```python
from build123d import *

# Parameters (mm, degrees)
SKETCH_1_W          = 40
SKETCH_1_H          = 37.5
EXTRUDE_1_DEPTH     = 19.9
SKETCH_2_W          = 7
SKETCH_2_H          = 19.9
EXTRUDE_2_DEPTH     = 2.5
CUT_EXTRUDE_1_DEPTH = 43.995581168


with BuildPart() as part:
    # 草图1 → 凸台-拉伸1 (new body)
    with BuildSketch(Plane.XY):
        Rectangle(SKETCH_1_W, SKETCH_1_H)
    extrude(amount=EXTRUDE_1_DEPTH)

    # 草图2 → 凸台-拉伸2 (add)
    with BuildSketch(Plane(origin=(0, 8.15, 0), x_dir=(-1, 0, 0), z_dir=(0, -1, 0))):
        with Locations((23.5, -9.95)):
            Rectangle(SKETCH_2_W, SKETCH_2_H)
        with Locations((-23.5, -9.95)):
            Rectangle(SKETCH_2_W, SKETCH_2_H)
    extrude(amount=EXTRUDE_2_DEPTH)

    # 草图3 → 切除-拉伸1 (cut, through all)
    with BuildSketch(Plane(origin=(0, 8.15, 0), x_dir=(1, 0, 0), z_dir=(0, 1, 0))):
        with BuildLine():
            Line((27, -15.9), (26.315564437, -15.9))
            ThreePointArc((26.315564437, -15.9), (22.05, -14.9), (26.315564437, -13.9))
            Line((26.315564437, -13.9), (27, -13.9))
            Line((27, -13.9), (27, -15.9))
        make_face()
        with BuildLine():
            Line((27, -6), (26.315564437, -6))
            ThreePointArc((26.315564437, -6), (22.05, -5), (26.315564437, -4))
            Line((26.315564437, -4), (27, -4))
            Line((27, -4), (27, -6))
        make_face()
        with BuildLine():
            Line((-27, -15.9), (-27, -13.9))
            Line((-27, -13.9), (-26.315564437, -13.9))
            ThreePointArc((-26.315564437, -13.9), (-22.05, -14.9), (-26.315564437, -15.9))
            Line((-26.315564437, -15.9), (-27, -15.9))
        make_face()
        with BuildLine():
            Line((-27, -4), (-27, -6))
            Line((-27, -6), (-26.315564437, -6))
            ThreePointArc((-26.315564437, -6), (-22.05, -5), (-26.315564437, -4))
            Line((-26.315564437, -4), (-27, -4))
        make_face()
    extrude(amount=-CUT_EXTRUDE_1_DEPTH, mode=Mode.SUBTRACT)


solid = part.part
```
Could you check a few things on this model? Use its own coordinates, in mm. A direction names the side the tool comes from. Coordinates: 2 decimals unless noted, no trailing zeros. Write each loop counter-clockwise with the first axis right and the second up, starting at its lowest first coordinate (ties: lowest second). Pieces come first, ordered by that corner, then holes. Notation, with made-up numbers: (45, 54.25) -> (104, 54.25) arc R24 cw to (104, 91.25) -> close; hole circle Ø2 at (1.5, -29.75). An arc over 180 degrees is marked (long way). Return JSON: item names as keys, results as strings.
(1) Imagine slicing it at A-A, the plane x = -24.3. Please give me the cut outline in (y, z).
Numbers:
{"outline": "(5.65, 0) -> (8.15, 0) -> (8.15, 2.75) -> (5.65, 2.75) -> close; (5.65, 7.25) -> (8.15, 7.25) -> (8.15, 12.65) -> (5.65, 12.65) -> close; (5.65, 17.15) -> (8.15, 17.15) -> (8.15, 19.9) -> (5.65, 19.9) -> close"}
(2) We'd pull the mould along X, two halves only. Please class faces 1 (the flat face through (27, 7, 18)), 2 (the cylindrical face through (-22.05, 6.92, 5.08)), 3 (the flat face through (-27, 7, 10)), 4 (the cylindrical face through (22.05, 6.92, 14.98)): +X half, -X half, draft (parallel to the pull), parting line (faces both ways), or undercut.
Numbers:
{"face 1": "+X half", "face 2": "undercut", "face 3": "-X half", "face 4": "undercut"}
(3) Imagine slicing it at B-B, the plane z = 5. Please give me the cut outline in (x, y), then the cut area to 3 significant figures.
Numbers:
{"outline": "(-22.05, 5.65) -> (-20, 5.65) -> (-20, -18.75) -> (20, -18.75) -> (20, 5.65) -> (22.05, 5.65) -> (22.05, 8.15) -> (20, 8.15) -> (20, 18.75) -> (-20, 18.75) -> (-20, 8.15) -> (-22.05, 8.15) -> close", "area": "1,510 mm2"}
(4) I'm going to push flat-ended pins straight in: pin 1 (3.5 mm diameter, centred on x = -23, z = 10, fed in from -Y); pin 2 (1.5 mm diameter, centred on y = 10.5, z = 4.5, fed in from +X); pin 3 (5 mm diameter, centred on x = -24.3, z = 5, fed in from +Y). Where does each tip first touch, or does it pass through?
Numbers:
{"pin 1": "stops at y = 5.65", "pin 2": "stops at x = 20", "pin 3": "stops at y = 8.15"}
(5) Which directions (+Z, -Z, +X, -X, +Y, -Y) give clear straight access to the entire face, cutting with the end or side of a thin tool? Please do faces 5 (the flat face through (24, 8.15, 10)), 6 (the flat face through (-20, -7, 10)), 7 (the flat face through (-20, 13, 10)).
Numbers:
{"face 5": "+Z, -Z, +X, +Y", "face 6": "+Z, -Z, -X, -Y", "face 7": "+Z, -Z, -X, +Y"}
(6) Imagine slicing it at C-C, the plane z = 16.5. Please give me the cut outline in (x, y).
Numbers:
{"outline": "(-27, 5.65) -> (-25.88, 5.65) -> (-25.88, 8.15) -> (-27, 8.15) -> close; (-22.72, 5.65) -> (-20, 5.65) -> (-20, -18.75) -> (20, -18.75) -> (20, 5.65) -> (22.72, 5.65) -> (22.72, 8.15) -> (20, 8.15) -> (20, 18.75) -> (-20, 18.75) -> (-20, 8.15) -> (-22.72, 8.15) -> close; (25.88, 5.65) -> (27, 5.65) -> (27, 8.15) -> (25.88, 8.15) -> close"}
(7) Imagine slicing it at D-D, the plane y = 11.5. Please give me the cut outline in (x, z).
Numbers:
{"outline": "(-20, 0) -> (20, 0) -> (20, 19.9) -> (-20, 19.9) -> close"}
(8) I need wall thicknesses on L1, parallel to Z at x = 24.3, y = 6.3; L2, parallel to X at y = 7.1, z = 14.9; L3, parallel to X at y = 11, z = 2.75. Which ranges of each line are inside material? Lowest first, please.
Numbers:
{"L1": "z = 0 to 2.75, 7.25 to 12.65, 17.15 to 19.9", "L2": "x = -22.05 to 22.05", "L3": "x = -20 to 20"}
